Geometry: final body of the model. Coordinates: model frame, mm. A direction names the side the tool comes from. Round coordinates to 2 decimals unless told otherwise and drop trailing zeros. Write each loop counter-clockwise with the first axis right and the second up, starting at its lowest first coordinate (ties: lowest second). Pieces come first, ordered by that corner, then holes. Notation, with made-up numbers: M 44.5,-32.5 L 65.5,-32.5 A15 cw 65.5,-8.5 Z; hole C -8,23 d5. An arc over 180 degrees is marked long. Use one line per item in the form item = value. Start each with the question number.
from build123d import *

# Parameters (mm, degrees)
PAD014_DEPTH    = 23
PAD015_DEPTH    = 23
SKETCH022_W     = 36
SKETCH022_H     = 23
PAD016_DEPTH    = 3
SKETCH023_R     = 1.4
POCKET004_DEPTH = 5


with BuildPart() as part:
    # Sketch019 → Pad014 (new body)
    with BuildSketch(Plane.XY):
        Polygon((4, 4), (42, 4), (42, 32), (37, 32), (37, 36), (46, 36), (46, 0), (0, 0), (0, 36), (9, 36), (9, 32), (4, 32), align=None)
    extrude(amount=PAD014_DEPTH)

    # Sketch020 → Pad015 (join)
    with BuildSketch(Plane.XY):
        with BuildLine():
            ThreePointArc((43.763932, -2), (48.738613, -1.224745), (46, 3))
            Line((46, 3), (46, 0))
            Line((0, 0), (46, 0))
            Line((0, 3), (0, 0))
            ThreePointArc((0, 3), (-2.738613, -1.224745), (2.236068, -2))
            Line((2.236068, -2), (43.763932, -2))
        make_face()
    extrude(amount=PAD015_DEPTH)

    # Sketch022 → Pad016 (join)
    with BuildSketch(Plane.YZ):
        with Locations((18, 11.5)):
            Rectangle(SKETCH022_W, SKETCH022_H)
    extrude(amount=-PAD016_DEPTH)

    # Sketch023 → Pocket004 (cut, symmetric)
    with BuildSketch(Plane.YZ):
        with Locations((7, 20)):
            Circle(SKETCH023_R)
        with Locations((24, 20)):
            Circle(SKETCH023_R)
        with Locations((7, 3)):
            Circle(SKETCH023_R)
        with Locations((24, 3)):
            Circle(SKETCH023_R)
    extrude(amount=POCKET004_DEPTH, both=True, mode=Mode.SUBTRACT)


solid = part.part
1. Contact query for flat-ended pins moving along their axis: pin 1 (3 mm diameter, centred on x = 35.5, z = 16.5, fed in from -Y); pin 2 (2.5 mm diameter, centred on y = 7, z = 20, fed in from +X); pin 3 (1.5 mm diameter, centred on x = 31.5, y = 5.5, fed in from +Z) (3 decimals); pin 4 (1.7 mm diameter, centred on y = 24, z = 3, fed in from -X). Output: stop coordinate, or through.
2. Set-up query: faces 1 (the face through (37, 34, 11)), 2 (the face through (40, 32, 11)), 3 (the face through (46, 20, 11)). Return all of +Z, -Z, +X, -X, +Y, -Y with unobstructed straight access to the full face (end or side cutting, diameter ignored); none if empty.
3. Section query A-A (y = 24). Return loops of the section in (x, z).
4. Ray query, probe 1 along Z at (x, y) = (1.5, 24); probe 2 along Y at (x, z) = (2.75, 20); probe 3 along X at (y, z) = (28.5, 9.75). Return the intervals inside material, ascending.
5. Section query C-C (z = 3). Return loops of the section in (x, y).
6. Pull-direction query (Z, two-part tool) for faces 4 (the face through (23, 4, 11)), 5 (the face through (0.549, 6.697, 1.633)), 6 (the face through (21, 3, 23)); classes: released by +Z, released by -Z, zero draft, split by the parting line, or undercut.
7. Section query D-D (y = 33). Return loops of the section in (x, z).
8. Section query B-B (x = 6.5). Return loops of the section in (y, z).
Checks:
q1.pin_1 = -2
q1.pin_2 = 46
q1.pin_3 = through
q1.pin_4 = 42
q2.face_1 = +Z, -Z, +Y
q2.face_2 = +Z, -Z
q2.face_3 = +Z, -Z, +X, +Y
q3.outline = M -3,0 L 4,0 L 4,1.6 L -3,1.6 Z; M -3,4.4 L 4,4.4 L 4,18.6 L -3,18.6 Z; M -3,21.4 L 4,21.4 L 4,23 L -3,23 Z; M 42,0 L 46,0 L 46,23 L 42,23 Z
q4.probe_1 = 0 to 1.6, 4.4 to 18.6, 21.4 to 23
q4.probe_2 = -2 to 5.6, 8.4 to 22.6, 25.4 to 36
q4.probe_3 = -3 to 4, 42 to 46
q5.outline = M -3,0 A3 ccw 2.24,-2 L 43.76,-2 A3 ccw long 46,3 L 46,36 L 37,36 L 37,32 L 42,32 L 42,4 L 4,4 L 4,5.6 L -3,5.6 Z; M -3,8.4 L 4,8.4 L 4,22.6 L -3,22.6 Z; M -3,25.4 L 4,25.4 L 4,32 L 9,32 L 9,36 L -3,36 Z
q6.face_4 = zero draft
q6.face_5 = undercut
q6.face_6 = released by +Z
q7.outline = M -3,0 L 9,0 L 9,23 L -3,23 Z; M 37,0 L 46,0 L 46,23 L 37,23 Z
q8.outline = M -2,0 L 4,0 L 4,23 L -2,23 Z; M 32,0 L 36,0 L 36,23 L 32,23 Z
